Here's how the part is built. I have some questions about the finished solid (model axes, mm). Face numbers are marked on the shaded views. A direction names the side the tool comes from. Coordinates: 2 decimals unless noted, no trailing zeros. Write each loop counter-clockwise with the first axis right and the second up, starting at its lowest first coordinate (ties: lowest second). Pieces come first, ordered by that corner, then holes.
(1) Imagine slicing it at A-A, the plane y = 5.1. List the corners of the cut face in (x, z) for me, plus the area to 3 significant figures.
(2) Imagine slicing it at D-D, the plane z = -8.5. List the corners of the cut face in (x, y) for me, plus the area to 3 significant figures.
(3) Imagine slicing it at B-B, the plane z = -13.75. List the corners of the cut face in (x, y) for me.
(4) Thinking about a two-plate mould opening in Z: for the marked faces 1, 2, 3 and 4, which applies, released by +Z, released by -Z, zero draft, split by the parting line, or undercut?
(5) Which directions (+Z, -Z, +X, -X, +Y, -Y) give clear straight access to the entire face, cutting with the end or side of a thin tool? Please do the marked faces 5, 6 and 7.
(6) Imagine slicing it at C-C, the plane x = -6. List the corners of the cut face in (y, z) for me.
(7) Please list where these lines run through material, in increasing order: probe 1 along Z at (x, y) = (-1.5, 4.35); probe 2 along X at (y, z) = (3.8, -14); probe 3 along Y at (x, z) = (-5, -1.75).
Autodesk Inventor part; units mm, degrees
ref_plane "РабПлоскость1" through (-10, 6, -7.5) normal (0, 0, 1) x (1, 0, 0)
ref_plane "YZ Plane" through (0, 0, 0) normal (1, 0, 0) x (0, 1, 0)
ref_plane "XZ Plane" through (0, 0, 0) normal (0, 1, 0) x (-1, 0, 0)
sketch "Эскиз1" plane through (0, 0, 0) normal (0, 1, 0) x (-1, 0, 0)
  line L0 (0, 0) -> (10, 0)
  line L1 (10, 0) -> (10, -15)
  line L2 (10, -15) -> (0, -15)
  line L3 (0, -15) -> (0, 0)
  dimension "d0" = 10
  dimension "d1" = 15
extrude "Выдавливание1" add sketch "Эскиз1" along normal blind 6
sketch "Эскиз2" plane through (0, 6, 0) normal (0, 1, 0) x (1, 0, 0)
  line L0 (-10, 15) -> (-10, 0)
  line L1 (-10, 0) -> (-10, 5)
  line L2 (0, 0) -> (0, 15)
  line L3 (-10, 5) -> (0, 5)
  line L4 (0, 5) -> (0, 10)
  line L5 (0, 10) -> (-10, 10)
  line L6 (-10, 10) -> (-10, 5)
  line L7 (-10, 10) -> (-10, 15)
  line L8 (-10, 0) -> (0, 0)
  point P0 (0, 5)
  dimension "d4" = 5
extrude "Выдавливание2" cut sketch "Эскиз2" against normal blind 3 contours L5 L2 L3 L0
sketch "Эскиз3" plane through (-10, 0, 0) normal (0, 0, 1) x (1, 0, 0)
  line L0 (2.45, 4) -> (7.55, 4)
  line L1 (7.55, 4) -> (7.55, 1.9)
  line L2 (7.55, 1.9) -> (2.45, 1.9)
  line L3 (2.45, 1.9) -> (2.45, 4)
  line L4 (2.45, 2.95) -> (0, 2.95)
  line L5 (0, 0) -> (0, 6)
  line L6 (7.55, 2.95) -> (10, 2.95)
  line L7 (10, 0) -> (10, 6)
  line L8 (5, 4) -> (5, 6)
  line L9 (10, 6) -> (0, 6)
  dimension "d7" = 5.1
  dimension "d8" = 2.1
  dimension "d12" = 2
extrude "Выдавливание3" cut sketch "Эскиз3" against normal blind 2.15 contours L0 L1 L2 L3
ref_plane "РабПлоскость1" through (-10, 6, -7.5) normal (0, 0, 1) x (1, 0, 0)
mirror "Зеркальное отражение1" about plane through (-10, 6, -7.5) normal (0, 0, 1) of "Выдавливание3"
chamfer "Фаска1" distance 2 angle 45 2 edges at (-5, 1.9, -2.15) (-5, 1.9, -12.85)
properties part number "Тестовая коробка"
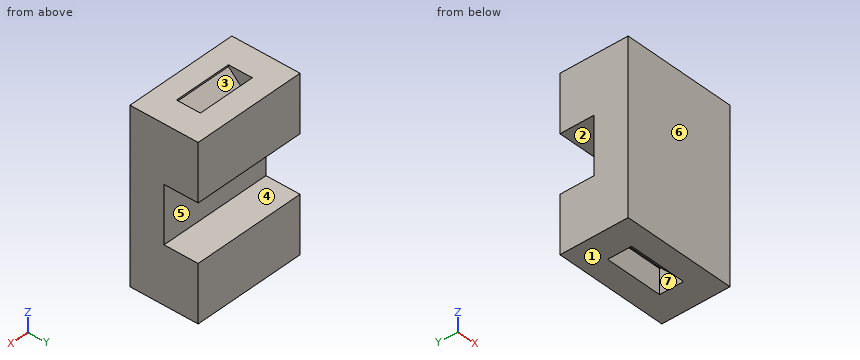
Recorded:
1. outline: (-10, -15) - (0, -15) - (0, -10) - (-10, -10) - close; (-10, -5) - (0, -5) - (0, 0) - (-10, 0) - close
1. area: 100 mm2
2. outline: (-10, 0) - (0, 0) - (0, 3) - (-10, 3) - close
2. area: 30.0 mm2
3. outline: (-10, 0) - (0, 0) - (0, 6) - (-10, 6) - close; hole (-7.55, 3) - (-2.45, 3) - (-2.45, 4) - (-7.55, 4) - close
4. face 1: released by -Z
4. face 2: undercut
4. face 3: released by +Z
4. face 4: undercut
5. face 5: +X, -X, +Y
5. face 6: +Z, -Z, +X, -X, -Y
5. face 7: -Z
6. outline: (0, -15) - (1.9, -15) - (1.9, -14.85) - (3.9, -12.85) - (4, -12.85) - (4, -15) - (6, -15) - (6, -10) - (3, -10) - (3, -5) - (6, -5) - (6, 0) - (4, 0) - (4, -2.15) - (3.9, -2.15) - (1.9, -0.15) - (1.9, 0) - (0, 0) - close
7. probe 1: z = -15 to -10, -5 to 0
7. probe 2: x = -10 to -7.55, -2.45 to 0
7. probe 3: y = 0 to 3.5, 4 to 6
